Verification items for the finished model (mm, model axes). A direction names the side the tool comes from. Coordinates: 2 decimals unless noted, no trailing zeros. Order: outer loops, then holes, each group sorted by start corner. A loop starts at its lowest first (then second) coordinate and runs counter-clockwise, first axis right, second up. Notation, with made-up numbers: (-14, 60.5) -> (23, 60.5) arc R18 cw to (23, 92.5) -> close; hole circle Ø8 at (66, -12). An arc over 180 degrees is marked (long way). Write item = value, one per line. Start each with the question number.
1. Cross-section at A-A on x = 23. Record the cut outline in (y, z), plus the area to 3 significant figures.
2. Set-up check for faces 1 (the flat face through (0, 2, 0)), 2 (the flat face through (13, 12, -7)), 3 (the cylindrical face through (13.3, 3.9, -13.5)): record each of +Z, -Z, +X, -X, +Y, -Y from which the full face is reachable in a straight line by a thin tool's end or side.
3. Cross-section at D-D on z = -0.5. Record the cut outline in (x, y), plus the area to 3 significant figures.
4. Cross-section at C-C on z = 11. Record the cut outline in (x, y), plus the area to 3 significant figures.
5. Cross-section at B-B on y = 4. Record the cut outline in (x, z), plus the area to 3 significant figures.
6. Release check for a two-part mould opening along Z. For faces 4 (the flat face through (13, 8, 11)), 5 (the cylindrical face through (13.3, 4.1, 13.5)), 6 (the cylindrical face through (12.72, 7.1, 14.14)) record: +Z half, -Z half, draft (parallel to the pull), parting line (faces both ways), or undercut.
7. Go/stop test with flat-tipped pins: P1, Ø4, axis at y = 4, z = 11, coming from the -X side; P2, Ø2.5, axis at x = 13.5, y = 12.5, coming from the -Z side; P3, Ø5.5, axis at x = 11, z = 2.5, coming from the +Y side; P4, Ø2, axis at x = 8.5, z = -11, coming from the +Y side. Record where each tip stops, or that it passes through.
8. Thickness scan on line 1 along Y through (x, z) = (5.5, -11); line 2 along Z through (x, y) = (-0.5, 5); line 3 along X through (y, z) = (12.5, 4.5). Record the ranges inside material, lowest first. Write a range as from..to.
Autodesk Inventor part; units mm, degrees
ref_plane "YZ Plane" through (0, 0, 0) normal (1, 0, 0) x (0, 1, 0)
ref_plane "XZ Plane" through (0, 0, 0) normal (0, 1, 0) x (-1, 0, 0)
ref_plane "XY Plane" through (0, 0, 0) normal (0, 0, 1) x (1, 0, 0)
sketch "Sketch1" plane through (0, 0, 0) normal (0, 1, 0) x (-1, 0, 0)
  line L0 (-7, 7) -> (7, 7)
  line L1 (7, 7) -> (7, -7)
  line L2 (7, -7) -> (-7, -7)
  line L3 (-7, -7) -> (-7, 7)
  line L4 (-7, 7) -> (7, -7) construction
  line L5 (7, 7) -> (-7, -7) construction
  point P0 (0, 0)
  dimension "d0" = 14
  dimension "d1" = 14
extrude "Extrusion1" add sketch "Sketch1" along normal blind 14
sketch "Sketch2" plane through (0, 14, 0) normal (0, 1, 0) x (1, 0, 0)
  line L0 (6, -6) -> (-6, -6)
  line L1 (-6, -6) -> (-6, 6)
  line L2 (-6, 6) -> (6, 6)
  line L3 (6, 6) -> (6, -6)
  line L4 (6, -6) -> (-6, 6) construction
  line L5 (-6, -6) -> (6, 6) construction
  point P0 (0, 0)
  dimension "d4" = 12
  dimension "d5" = 12
extrude "Extrusion2" cut sketch "Sketch2" against normal blind 12 draft -2
pattern_linear "Rectangular Pattern1" count 3 spacing 13 along (1, 0, 0) of "Extrusion2", "Extrusion1"
sketch "Sketch3" plane through (33, 0, 7) normal (1, 0, 0) x (0, 0, -1)
  line L0 (0, 0) -> (0, 14)
  line L1 (0, 0) -> (-8, 0)
  line L2 (-8, 0) -> (-8, 8)
  line L3 (-8, 8) -> (0, 8)
  line L4 (0, 8) -> (0, 0)
  line L5 (-4, 8) -> (-4, 0) construction
  circle A0 centre (-4, 4) radius 2.5
  point P0 (7, 0)
  dimension "d11" = 8
  dimension "d12" = 8
  dimension "d13" = 5
extrude "Extrusion3" add sketch "Sketch3" against normal up to surface (40 mm away)
fillet "Fillet1" radius 3 2 edges at (13, 8, 15) (13, 8, 7)
mirror "Mirror1" about plane through (0, 0, 0) normal (0, 0, 1) of "Fillet1", "Extrusion3"
fillet_without_effect "Fillet2"
properties part number "Mould"
Worked out:
q1.outline = (0, -15) -> (5, -15) arc R3 ccw to (8, -12) -> (8, -10) arc R3 cw to (11, -7) -> (14, -7) -> (14, -6) -> (2, -5.58) -> (2, 5.58) -> (14, 6) -> (14, 7) -> (11, 7) arc R3 cw to (8, 10) -> (8, 12) arc R3 ccw to (5, 15) -> (0, 15) -> close; hole circle Ø5 at (4, -11); hole circle Ø5 at (4, 11)
q1.area = 146 mm²
q2.face_1 = +Y
q2.face_2 = -Z, +X, -X, +Y
q2.face_3 = +X, -X
q3.outline = (-7, 0) -> (33, 0) -> (33, 14) -> (32, 14) -> (31.58, 2) -> (20.42, 2) -> (20, 14) -> (19, 14) -> (18.58, 2) -> (7.42, 2) -> (7, 14) -> (6, 14) -> (5.58, 2) -> (-5.58, 2) -> (-6, 14) -> (-7, 14) -> close
q3.area = 143 mm²
q4.outline = (-7, 0) -> (33, 0) -> (33, 1.5) -> (-7, 1.5) -> close; (-7, 6.5) -> (33, 6.5) -> (33, 8) -> (-7, 8) -> close
q4.area = 120 mm²
q5.outline = (-7, -15) -> (33, -15) -> (33, -13.5) -> (-7, -13.5) -> close; (-7, -8.5) -> (33, -8.5) -> (33, 8.5) -> (-7, 8.5) -> close; (-7, 13.5) -> (33, 13.5) -> (33, 15) -> (-7, 15) -> close; hole (-5.65, -5.65) -> (5.65, -5.65) -> (5.65, 5.65) -> (-5.65, 5.65) -> close; hole (7.35, -5.65) -> (18.65, -5.65) -> (18.65, 5.65) -> (7.35, 5.65) -> close; hole (20.35, -5.65) -> (31.65, -5.65) -> (31.65, 5.65) -> (20.35, 5.65) -> close
q5.area = 417 mm²
q6.face_4 = draft
q6.face_5 = undercut
q6.face_6 = +Z half
q7.P1 = through
q7.P2 = -7
q7.P3 = 2
q7.P4 = 8
q8.line_1 = 0..1.5, 6.5..8
q8.line_2 = -15..-13.29, -8.71..-5.69, 5.69..8.71, 13.29..15
q8.line_3 = -7..-5.95, 5.95..7.05, 18.95..20.05, 31.95..33
